from build123d import *

# Parameters (mm, degrees)
F0_R     = 18.875359
F1_DEPTH = 25.4
F2_DEPTH = 10.16
F3_R     = 25.4


with BuildPart() as f1:
    # F0 (on Top) → F1 (new body)
    with BuildSketch(Plane.XY):
        with BuildLine():
            Line((-23.921628, 15.438856), (-28.302625, 3.09257))
            ThreePointArc((-28.302625, 3.09257), (-2.154046, -28.389482), (28.445225, -1.213161))
            Line((28.445225, -1.213161), (22.189711, 17.838703))
            ThreePointArc((22.189711, 17.838703), (12.302751, 25.675764), (0, 28.471083))
            ThreePointArc((0, 28.471083), (-13.620602, 25.001635), (-23.921628, 15.438856))
        make_face()
        Circle(F0_R, mode=Mode.SUBTRACT)
    extrude(amount=F1_DEPTH)

    # F0 (on Top) → F2 (join)
    with BuildSketch(Plane.XY):
        with BuildLine():
            Line((-23.921628, 15.438856), (-28.302625, 3.09257))
            ThreePointArc((-28.302625, 3.09257), (-2.154046, -28.389482), (28.445225, -1.213161))
            Line((28.445225, -1.213161), (22.189711, 17.838703))
            ThreePointArc((22.189711, 17.838703), (12.302751, 25.675764), (0, 28.471083))
            ThreePointArc((0, 28.471083), (-13.620602, 25.001635), (-23.921628, 15.438856))
        make_face()
        Circle(F0_R, mode=Mode.SUBTRACT)
        with BuildLine():
            Line((-9.555586, 55.924454), (-23.921628, 15.438856))
            ThreePointArc((-23.921628, 15.438856), (-13.620602, 25.001635), (0, 28.471083))
            Line((0, 28.471083), (0, 47.159142))
            ThreePointArc((0, 47.159142), (-6.483439, 49.682373), (-9.555586, 55.924454))
        make_face()
        with BuildLine():
            ThreePointArc((0, 28.471083), (12.302751, 25.675764), (22.189711, 17.838703))
            Line((22.189711, 17.838703), (9.578088, 56.248801))
            ThreePointArc((9.578088, 56.248801), (6.602304, 49.793277), (0, 47.159142))
            Line((0, 47.159142), (0, 28.471083))
        make_face()
        with BuildLine():
            ThreePointArc((4.935129, 56.750353), (-3.489663, 60.240017), (0, 51.815224))
            ThreePointArc((0, 51.815224), (3.489663, 53.26069), (4.935129, 56.750353))
        make_face()
        with BuildLine():
            ThreePointArc((9.591211, 56.750353), (-0.413334, 66.332654), (-9.555586, 55.924454))
            ThreePointArc((-9.555586, 55.924454), (-6.483439, 49.682373), (0, 47.159142))
            ThreePointArc((0, 47.159142), (6.602304, 49.793277), (9.578088, 56.248801))
            ThreePointArc((9.578088, 56.248801), (9.58793, 56.499491), (9.591211, 56.750353))
        make_face()
        with BuildLine():
            ThreePointArc((4.935129, 56.750353), (3.489663, 53.26069), (0, 51.815224))
            ThreePointArc((0, 51.815224), (-3.489663, 60.240017), (4.935129, 56.750353))
        make_face(mode=Mode.SUBTRACT)
    extrude(amount=F2_DEPTH)

    # F3
    f3_edges = [f1.edges().sort_by_distance(p)[0] for p in [
        (22.189711, 17.838703, 17.78),
        (28.445225, -1.213161, 12.7),
        (9.578088, 56.248801, 5.08),
        (-9.555586, 55.924454, 5.08),
        (-28.302625, 3.09257, 12.7),
        (-23.921628, 15.438856, 17.78),
    ]]
    fillet(f3_edges, radius=F3_R)


solid = f1.part
Can you work these out from the model? Positions are in its coordinate system, mm. A direction names the side the tool comes from. Coordinates: 2 decimals unless noted, no trailing zeros. Loops run counter-clockwise (first coordinate to the right, second up) from the corner with the lowest first, then second, coordinate; pieces in that order, holes last. Notation, with made-up numbers: (25, 14) - (55, 14) arc R30 cw to (55, 49) - close; hole circle Ø9 at (4, 67.5). An arc over 180 degrees is marked (long way). Answer as a JSON object with one key per item and string values. Group by question number.
Item 1: If we section it at C-C (y = 0): List the corners of the cut face in (x, z) for me, plus the area to 3 significant figures.
Item 2: If we section it at A-A (x = -15): List the corners of the cut face in (y, z) for me.
Item 3: On a 3-axis mill with a long thin cutter (end or side, diameter ignored), from which of +Z, -Z, +X, -X, +Y, -Y can I reach the whole of each face in a straight line? I mean faces 5 (the face through (-20.984, 18.973, 17.887)), 6 (the face through (-10.004, 55.143, 5.151)), 7 (the face through (16.386, 22.72, 17.887)). Say none if no direction works.
Item 4: If we section it at B-B (z = 20.25): List the corners of the cut face in (x, y) for me, plus the area to 3 significant figures.
Item 5: If we mould it in two halves opening along X, with no side actions, what happens to faces 1 (the face through (-28.25, -1.5, 12.88)), 2 (the face through (-19.4, 0.4, 25.4)), 3 (the face through (26.56, -8.98, 12.88)), 4 (the face through (-4.092, -18.427, 12.522))? For each: released by +X, released by -X, zero draft, split by the parting line, or undercut.
Item 6: If I drill on L1, parallel to Y at x = 0, z = 4; L2, parallel to Y at x = 0, z = 15.75; L3, parallel to Y at x = -4.5, z = 4.5, over which ranges is the centre line in solid material (lowest first)? Write a range as from..to.
Item 7: If we section it at D-D (z = 4.25): State how many separate pieces and enclosed holes the cut face has, plus the area to 3 significant figures.
Item 8: For pin 1 (15 mm diameter, centred on x = -2, y = 43, fed in from +Z); pin 2 (2 mm diameter, centred on x = -12.5, z = 22, fed in from +Y); pin 3 (1 mm diameter, centred on x = 10, z = 8, fed in from -Y); pin 4 (8 mm diameter, centred on x = 0, y = 56.75, fed in from -Z), each with a flat end and sliding along its axis, tell me the tip position at first contact or that it passes through.
Returned:
{
 "1": {"outline": "(-28.23, 0) - (-18.88, 0) - (-18.88, 25.4) - (-28.23, 25.4) - close; (18.88, 0) - (27.36, 0) - (27.36, 25.4) - (18.88, 25.4) - close", "area": "453 mm²"},
 "2": {"outline": "(-24.2, 0) - (-11.46, 0) - (-11.46, 25.4) - (-24.2, 25.4) - close; (11.46, 0) - (40.58, 0) - (40.58, 10.16) - (24.19, 10.16) - (24.19, 25.4) - (11.46, 25.4) - close"},
 "3": {"face 5": "+Z, -X, +Y", "face 6": "+Z, -Z, -X, +Y", "face 7": "+Z, +X, +Y"},
 "4": {"outline": "(-26.79, 7.36) arc R25.4 ccw to (-26.44, -10.55) arc R28.47 ccw to (19.1, -21.11) arc R25.4 ccw to (26.19, 5.65) - (24.44, 10.98) arc R25.4 ccw to (2.87, 28.33) arc R28.47 ccw to (0, 28.47) arc R28.47 ccw to (-13.88, 24.86) arc R25.4 ccw to (-25.43, 11.18) - close; hole circle Ø37.75 at (0, 0)", "area": "1,370 mm²"},
 "5": {"face 1": "released by -X", "face 2": "zero draft", "face 3": "released by +X", "face 4": "undercut"},
 "6": {"L1": "y = -28.47..-18.88, 18.88..51.82, 61.69..66.34", "L2": "y = -28.47..-18.88, 18.88..28.47", "L3": "y = -28.11..-18.33, 18.33..54.72, 58.78..65.22"},
 "7": {"separate pieces": "1", "enclosed holes": "2", "area": "2,370 mm²"},
 "8": {"pin 1": "stops at z = 10.16", "pin 2": "stops at y = 26.05", "pin 3": "stops at y = -26.84", "pin 4": "passes through"}
}
